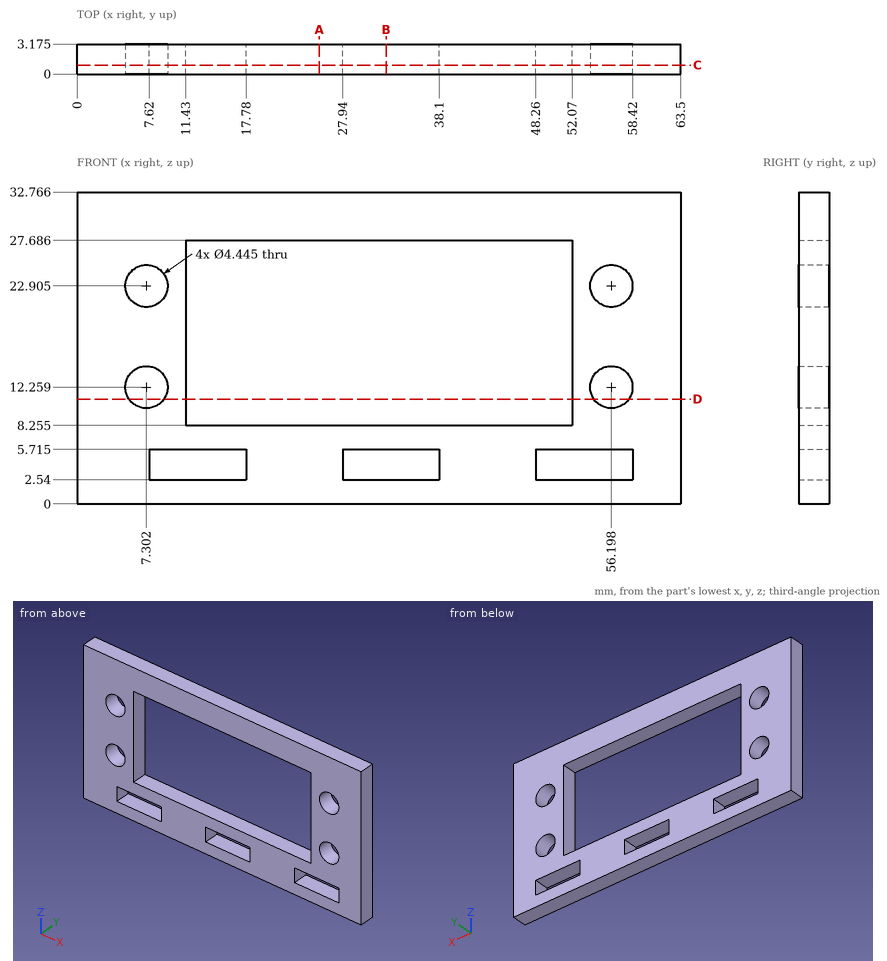
Design review of the part shown in the three views and the two pictorial views. Dimensions are in mm from the part's minimum x, y and z. Coordinates: 2 decimals unless noted, no trailing zeros. Loops run counter-clockwise (first coordinate to the right, second up) from the corner with the lowest first, then second, coordinate; pieces in that order, holes last. Notation, with made-up numbers: M 81.25,65.25 L 105.25,65.25 A15 ccw 105.25,90.25 Z; hole C 80.5,1.25 d10. An arc over 180 degrees is marked long. Put each result on its own line as item: value. Start each with the question number.
Q1. Add section D-D (z = 11). Write out the cut boundary in (x, y) (1 decimal).
Q2. Wall thickness on line 1 (Z direction, x = 12.5, y = 1.7) (1 decimal); line 2 (X direction, y = 2.3, z = 4); line 3 (X direction, y = 0.2, z = 18.5): over which ranges is each line inside the solid? List them lowest first.
Q3. Add section A-A (x = 25.5). Write out the cut boundary in (y, z) (1 decimal).
Q4. Add section B-B (x = 32.5). Write out the cut boundary in (y, z) (1 decimal).
Q5. Add section C-C (y = 0.95). Count the separate pieces of the cut face and the enclosed holes in it, and give its area (3 significant figures).
Answers:
1. outline: M 0,0 L 5.5,0 L 5.5,3.2 L 0,3.2 Z; M 9.1,0 L 11.4,0 L 11.4,3.2 L 9.1,3.2 Z; M 52.1,0 L 54.4,0 L 54.4,3.2 L 52.1,3.2 Z; M 58,0 L 63.5,0 L 63.5,3.2 L 58,3.2 Z
2. line 1: z = 0 to 2.5, 5.7 to 8.3, 27.7 to 32.8
2. line 2: x = 0 to 7.62, 17.78 to 27.94, 38.1 to 48.26, 58.42 to 63.5
2. line 3: x = 0 to 11.43, 52.07 to 63.5
3. outline: M 0,0 L 3.2,0 L 3.2,8.3 L 0,8.3 Z; M 0,27.7 L 3.2,27.7 L 3.2,32.8 L 0,32.8 Z
4. outline: M 0,0 L 3.2,0 L 3.2,2.5 L 0,2.5 Z; M 0,5.7 L 3.2,5.7 L 3.2,8.3 L 0,8.3 Z; M 0,27.7 L 3.2,27.7 L 3.2,32.8 L 0,32.8 Z
5. separate pieces: 1
5. enclosed holes: 8
5. area: 1,130 mm^2
